Could you check a few things on this model? Use its own coordinates, in mm. A direction names the side the tool comes from. Give positions to 0.01 mm unless a question says otherwise; leave off trailing zeros. Order: outer loops, then holes, each group sorted by start corner. A loop starts at its lowest first (then second) coordinate and runs counter-clockwise, first axis right, second up. Notation, with made-up numbers: M -27.75,-13.5 L -12.75,-13.5 A18 ccw -12.75,0.5 Z; hole C 54.25,83 d8. An arc over 180 degrees is marked long. Use a Markdown table: item, result. Add a question column.
Item 1: Suppose I cut it at D-D on x = 16.5. Write out the boundary of the cut face in (y, z).
Item 2: Suppose I cut it at C-C on y = 17. Write out the boundary of the cut face in (x, z).
Item 3: I'm going to push flat-ended pins straight in: pin 1 Ø12 at (x, z) = (38.5, 104) entering from +Y; pin 2 Ø6.5 at (y, z) = (-6, 103.5) entering from -X; pin 3 Ø6.5 at (y, z) = (-3.5, 92) entering from +X; pin 4 Ø8 at (x, y) = (30, 3) entering from +Z. Where does each tip first touch, or does it pass through?
Item 4: For faces 4 (the face through (51, 23, 49)), 5 (the face through (8.026, -2.958, 7.352)), 6 (the face through (0, -4, 101)), 7 (the face through (25, 42, 24)), 8 (the face through (50, -4, 101)), which set-ups out of +Z, -Z, +X, -X, +Y, -Y let a thin tool reach every point of the face, with its end or its side?
Item 5: Suppose I cut it at A-A on x = 9.5. Write out the boundary of the cut face in (y, z).
Item 6: If I drill on L1, parallel to Z at x = 9.5, y = -4.6; L2, parallel to X at y = 38, z = 34; L3, parallel to Z at x = 25, y = -4.75, over which ranges is the centre line in solid material (lowest first)? Write a range as from..to.
Item 7: If we mould it in two halves opening along X, with no side actions, what happens to faces 1 (the face through (0, 21, 52)), 2 (the face through (25, -4, 150)), 3 (the face through (53, 18, 25))? For each: released by +X, released by -X, zero draft, split by the parting line, or undercut.
Item 8: Suppose I cut it at B-B on z = 6. Write out the boundary of the cut face in (x, y).
from build123d import *

# Parameters (mm, degrees)
F0_W      = 50
F0_H      = 150
F0_R      = 2
F0_R_2    = 11.5
F1_DEPTH  = 8
F2_SIZE   = 2
F3_W      = 50
F3_H      = 53
F4_DEPTH  = 3
F5_W      = 50
F5_H      = 53
F6_DEPTH  = 3
F7_W      = 56
F7_H      = 50
F8_DEPTH  = 3
F9_W      = 56
F9_H      = 56
F10_DEPTH = 3
F11_R     = 1
F13_DEPTH = 45


with BuildPart() as f1:
    # F0 (on Front) → F1 (new body)
    with BuildSketch(Plane.XZ):
        with Locations((25, 75)):
            Rectangle(F0_W, F0_H)
        with Locations((9.5, 6)):
            Circle(F0_R, mode=Mode.SUBTRACT)
        with Locations((9.5, 37)):
            Circle(F0_R, mode=Mode.SUBTRACT)
        with Locations((25, 21.5)):
            Circle(F0_R_2, mode=Mode.SUBTRACT)
        with Locations((40.5, 6)):
            Circle(F0_R, mode=Mode.SUBTRACT)
        with Locations((40.5, 37)):
            Circle(F0_R, mode=Mode.SUBTRACT)
    extrude(amount=F1_DEPTH)

    # F2
    f2_edges = [f1.edges().sort_by_distance(p)[0] for p in [
        (7.5, -8, 37),
        (38.5, -8, 37),
        (38.5, -8, 6),
        (7.5, -8, 6),
    ]]
    chamfer(f2_edges, length=F2_SIZE)

    # F3 (on face) → F4 (join)
    with BuildSketch(Plane.YZ.offset(50)):
        with Locations((17, 26.5)):
            Rectangle(F3_W, F3_H)
    extrude(amount=F4_DEPTH)

    # F5 (on face) → F6 (join)
    with BuildSketch(Plane(origin=(0, 0, 0), x_dir=(0, -1, 0), z_dir=(-1, 0, 0))):
        with Locations((-17, 26.5)):
            Rectangle(F5_W, F5_H)
    extrude(amount=F6_DEPTH)

    # F7 (on face) → F8 (join)
    with BuildSketch(Plane(origin=(0, 0, 0), x_dir=(1, 0, 0), z_dir=(0, 0, -1))):
        with Locations((25, -17)):
            Rectangle(F7_W, F7_H)
    extrude(amount=F8_DEPTH)

    # F9 (on face) → F10 (join)
    with BuildSketch(Plane(origin=(0, 42, 0), x_dir=(-1, 0, 0), z_dir=(0, 1, 0))):
        with Locations((-25, 25)):
            Rectangle(F9_W, F9_H)
    extrude(amount=F10_DEPTH)

    # F11
    f11_edges = [f1.edges().sort_by_distance(p)[0] for p in [
        (50, 0, 26.5),
        (25, 0, 0),
        (50, 21, 0),
        (0, 21, 0),
        (0, 42, 26.5),
        (50, 42, 26.5),
        (0, 0, 26.5),
        (25, 42, 0),
        (53, 45, 25),
        (25, 45, 53),
        (25, 45, -3),
        (-3, 45, 25),
        (25, -8, -3),
        (-3, 18.5, -3),
        (53, 18.5, -3),
        (53, -8, 25),
        (53, 18.5, 53),
        (-3, -8, 25),
        (-3, 18.5, 53),
    ]]
    fillet(f11_edges, radius=F11_R)

    # F12 (on face) → F13 (cut, through all)
    with BuildSketch(Plane(origin=(0, 45, 0), x_dir=(-1, 0, 0), z_dir=(0, 1, 0))):
        Polygon((-50, 50.1), (-51, 50.1), (-51, 47), (1, 47), (1, 50.1), (-1, 50.1), (-1, 53), (-50, 53), align=None)
    extrude(amount=-F13_DEPTH, mode=Mode.SUBTRACT)


solid = f1.part
Findings below:
| question | item | result |
|---|---|---|
| 1 | outline | M -8,-2 A1 ccw -7,-3 L 44,-3 A1 ccw 45,-2 L 45,47 L 42,47 L 42,1 A1 cw 41,0 L 1,0 A1 cw 0,1 L 0,13.75 L -8,13.75 Z; M -8,29.25 L 0,29.25 L 0,150 L -8,150 Z |
| 2 | outline | M -3,-2 A1 ccw -2,-3 L 52,-3 A1 ccw 53,-2 L 53,52 A1 ccw 52,53 L 50,53 L 50,50.1 L 51,50.1 L 51,47 L 50,47 L 50,1 A1 cw 49,0 L 1,0 A1 cw 0,1 L 0,47 L -1,47 L -1,50.1 L 0,50.1 L 0,53 L -2,53 A1 ccw -3,52 Z |
| 3 | pin 1 | stops at y = 0 |
| 3 | pin 2 | stops at x = 0 |
| 3 | pin 3 | stops at x = 50 |
| 3 | pin 4 | stops at z = 150 |
| 4 | face 4 | +Y |
| 4 | face 5 | -Y |
| 4 | face 6 | +Z, -X, +Y, -Y |
| 4 | face 7 | +Z |
| 4 | face 8 | +Z, +X, +Y, -Y |
| 5 | outline | M -8,-2 A1 ccw -7,-3 L 44,-3 A1 ccw 45,-2 L 45,47 L 42,47 L 42,1 A1 cw 41,0 L 1,0 A1 cw 0,1 L 0,4 L -6,4 L -8,2 Z; M -8,10 L -6,8 L 0,8 L 0,35 L -6,35 L -8,33 Z; M -8,41 L -6,39 L 0,39 L 0,150 L -8,150 Z |
| 6 | L1 | z = -3..4, 8..35, 39..150 |
| 6 | L2 | x = -3..0, 50..53 |
| 6 | L3 | z = -3..10, 33..150 |
| 7 | face 1 | undercut |
| 7 | face 2 | zero draft |
| 7 | face 3 | released by +X |
| 8 | outline | M -3,-7 A1 ccw -2,-8 L 5.5,-8 L 7.5,-6 L 7.5,0 L 1,0 A1 cw 0,1 L 0,41 A1 cw 1,42 L 49,42 A1 cw 50,41 L 50,1 A1 cw 49,0 L 42.5,0 L 42.5,-6 L 44.5,-8 L 52,-8 A1 ccw 53,-7 L 53,44 A1 ccw 52,45 L -2,45 A1 ccw -3,44 Z; M 11.5,-6 L 13.5,-8 L 36.5,-8 L 38.5,-6 L 38.5,0 L 11.5,0 Z |
